Read the model definition and answer for the solid it produces. Units are mm, in the model's axes. A direction names the side the tool comes from. Round coordinates to 2 decimals unless told otherwise and drop trailing zeros. Loops run counter-clockwise (first coordinate to the right, second up) from the corner with the lowest first, then second, coordinate; pieces in that order, holes last. Notation, with made-up numbers: (26, -15.75) - (30, -15.75) arc R26 ccw to (30, 16.25) - close; hole circle Ø10 at (8.25, 10.5). An arc over 180 degrees is marked (long way). Use CSV: the item, a comma, the result in double quotes. Start each with the question number.
1. Given pin 1 Ø1.5 at (x, z) = (0.5, 0.5) entering from -Y; pin 2 Ø4.5 at (x, y) = (-24.5, 0) entering from +Z, each flat-ended and moving along its own axis, determine where each tip first touches the part or whether it passes through.
2. A tool of negligible diameter and unlimited length cuts with its end or side. For faces 1 (the cylindrical face through (20.5, -6.6, 1.5)), 2 (the cylindrical face through (-28.93, -8.95, 1.52)), 3 (the cylindrical face through (-13.82, -9.433, 1.521)), from which of +Z, -Z, +X, -X, +Y, -Y can it reach the whole face along a straight path? Write none if from no direction.
3. Find section C-C (y = -5). Give the vertices of the cut face in (x, z).
4. Find section D-D (z = 2.4). State how many separate pieces and enclosed holes the cut face has, and give its area (3 significant figures).
5. Find section B-B (x = -24.5). Give the vertices of the cut face in (y, z), and give its area (4 significant figures).
6. Find section A-A (y = 0). Give the vertices of the cut face in (x, z), and give its area (3 significant figures).
7. Consider line 1 along X through (y, z) = (-5.5, 1.35); line 2 along Y through (x, z) = (-8, 0.65); line 3 along Y through (x, z) = (-24.5, 1.35). Determine where each line is inside the solid, lowest interval first.
8. Determine the mould class of faces 4 (the flat face through (0, 4, 1)), 5 (the flat face through (-29.5, -3, 1)), 6 (the cylindrical face through (-14.5, -6.6, 1.5)), 7 (the cylindrical face through (8.965, -5.674, 1.521)) for opening direction X: +X half, -X half, draft (parallel to the pull), parting line (faces both ways), or undercut.
from build123d import *

# Parameters (mm, degrees)
SKETCH_1_R      = 2.85
SKETCH_1_R_2    = 1.5
EXTRUDE_1_DEPTH = 3
FILLET_1_R      = 2


with BuildPart() as part:
    # 草图1 → 凸台-拉伸1 (new body)
    with BuildSketch(Plane.XY):
        Polygon((29.5, 4), (-29.5, 4), (-29.5, -9.55), (-13.76701437, -9.55), (-9, -5.55), (9, -5.55), (13.76701437, -9.55), (29.5, -9.55), align=None)
        with BuildLine():
            Line((-15.6, -5.55), (-19.4, -5.55))
            ThreePointArc((-19.4, -5.55), (-20.45, -6.6), (-21.5, -5.55))
            Line((-21.5, -5.55), (-21.5, -2.45))
            ThreePointArc((-21.5, -2.45), (-20.45, -1.4), (-19.4, -2.45))
            Line((-19.4, -2.45), (-15.6, -2.45))
            ThreePointArc((-15.6, -2.45), (-14.55, -1.4), (-13.5, -2.45))
            Line((-13.5, -2.45), (-13.5, -5.55))
            ThreePointArc((-13.5, -5.55), (-14.55, -6.6), (-15.6, -5.55))
        make_face(mode=Mode.SUBTRACT)
        with BuildLine():
            Line((13.5, -5.55), (13.5, -2.45))
            ThreePointArc((13.5, -2.45), (14.55, -1.4), (15.6, -2.45))
            Line((15.6, -2.45), (19.4, -2.45))
            ThreePointArc((19.4, -2.45), (20.45, -1.4), (21.5, -2.45))
            Line((21.5, -2.45), (21.5, -5.55))
            ThreePointArc((21.5, -5.55), (20.45, -6.6), (19.4, -5.55))
            Line((19.4, -5.55), (15.6, -5.55))
            ThreePointArc((15.6, -5.55), (14.55, -6.6), (13.5, -5.55))
        make_face(mode=Mode.SUBTRACT)
        with Locations((-24.5, 0)):
            Circle(SKETCH_1_R, mode=Mode.SUBTRACT)
        with Locations((-8, 0)):
            Circle(SKETCH_1_R_2, mode=Mode.SUBTRACT)
        with Locations((8, 0)):
            Circle(SKETCH_1_R_2, mode=Mode.SUBTRACT)
        with Locations((24.5, 0)):
            Circle(SKETCH_1_R, mode=Mode.SUBTRACT)
    extrude(amount=EXTRUDE_1_DEPTH)

    # 圆角1
    fillet_1_edges = [part.edges().sort_by_distance(p)[0] for p in [
        (9, -5.55, 1.5),
        (-9, -5.55, 1.5),
        (-13.76701437, -9.55, 1.5),
        (-29.5, -9.55, 1.5),
        (-29.5, 4, 1.5),
        (29.5, 4, 1.5),
        (29.5, -9.55, 1.5),
        (13.76701437, -9.55, 1.5),
    ]]
    fillet(fillet_1_edges, radius=FILLET_1_R)


solid = part.part
Filled sheet:
1,pin 1,"stops at y = -5.55"
1,pin 2,"passes through"
2,face 1,"+Z, -Z"
2,face 2,"+Z, -Z, -X, -Y"
2,face 3,"+Z, -Z, -Y"
3,outline,"(-29.5, 0) - (-21.5, 0) - (-21.5, 3) - (-29.5, 3) - close; (-13.5, 0) - (13.5, 0) - (13.5, 3) - (-13.5, 3) - close; (21.5, 0) - (29.5, 0) - (29.5, 3) - (21.5, 3) - close"
4,separate pieces,"1"
4,enclosed holes,"6"
4,area,"576 mm²"
5,outline,"(-9.55, 0) - (-2.85, 0) - (-2.85, 3) - (-9.55, 3) - close; (2.85, 0) - (4, 0) - (4, 3) - (2.85, 3) - close"
5,area,"23.55 mm²"
6,outline,"(-29.5, 0) - (-27.35, 0) - (-27.35, 3) - (-29.5, 3) - close; (-21.65, 0) - (-9.5, 0) - (-9.5, 3) - (-21.65, 3) - close; (-6.5, 0) - (6.5, 0) - (6.5, 3) - (-6.5, 3) - close; (9.5, 0) - (21.65, 0) - (21.65, 3) - (9.5, 3) - close; (27.35, 0) - (29.5, 0) - (29.5, 3) - (27.35, 3) - close"
6,area,"125 mm²"
7,line 1,"x = -29.5 to -21.5, -13.5 to 13.5, 21.5 to 29.5"
7,line 2,"y = -5.55 to -1.5, 1.5 to 4"
7,line 3,"y = -9.55 to -2.85, 2.85 to 4"
8,face 4,"draft"
8,face 5,"-X half"
8,face 6,"undercut"
8,face 7,"undercut"
